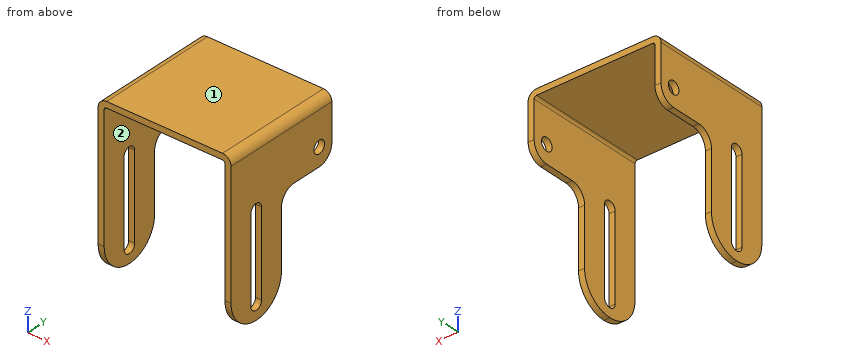
```python
from build123d import *

# Parameters (mm, degrees)
BASE_FLANGE1_DEPTH = 40
SKETCH6_W          = 34
SKETCH6_H          = 20
CUT_EXTRUDE1_DEPTH = 79.993670633
FILLET1_R          = 10
FILLET2_R          = 5
SKETCH7_R          = 2.1
CUT_EXTRUDE2_DEPTH = 79.993670633


# Read off the part's stored shape, not the designer's step: Base-Flange1
with BuildPart() as part:
    # Base-Flange1 outline → Base-Flange1 (new body)
    with BuildSketch(Plane(origin=(0, 0, 0), x_dir=(1, 0, 0), z_dir=(0, 1, 0))):
        with BuildLine():
            Line((-20, 0.8), (-20, 52))
            Line((-20, 52), (-22, 52))
            Line((-22, 52), (-22, 0.8))
            ThreePointArc((-22, 0.8), (-21.179898987, -1.179898987), (-19.2, -2))
            Line((-19.2, -2), (19.2, -2))
            ThreePointArc((19.2, -2), (21.179898987, -1.179898987), (22, 0.8))
            Line((22, 0.8), (22, 52))
            Line((22, 52), (20, 52))
            Line((20, 52), (20, 0.8))
            ThreePointArc((20, 0.8), (19.765685425, 0.234314575), (19.2, 0))
            Line((19.2, 0), (-19.2, 0))
            ThreePointArc((-19.2, 0), (-19.765685425, 0.234314575), (-20, 0.8))
        make_face()
    extrude(amount=BASE_FLANGE1_DEPTH)

    # Sketch6 → Cut-Extrude1 (cut, through all)
    with BuildSketch(Plane(origin=(22, 0, 0), x_dir=(0, 0, -1), z_dir=(1, 0, 0))):
        with Locations((35, 30)):
            Rectangle(SKETCH6_W, SKETCH6_H)
    extrude(amount=-CUT_EXTRUDE1_DEPTH, mode=Mode.SUBTRACT)

    # Fillet1
    fillet1_edges = [part.edges().sort_by_distance(p)[0] for p in [
        (-21, 0, -52),
        (-21, 20, -52),
        (21, 0, -52),
        (21, 20, -52),
    ]]
    fillet(fillet1_edges, radius=FILLET1_R - 0.0001)  # a hair under: the kernel refuses the full size

    # Fillet2
    fillet2_edges = [part.edges().sort_by_distance(p)[0] for p in [
        (-21, 40, -18),
        (21, 40, -18),
        (-21, 20, -18),
        (21, 20, -18),
    ]]
    fillet(fillet2_edges, radius=FILLET2_R)

    # Sketch7 → Cut-Extrude2 (cut, through all)
    with BuildSketch(Plane(origin=(22, 0, 0), x_dir=(0, 0, -1), z_dir=(1, 0, 0))):
        with Locations((12, 35)):
            Circle(SKETCH7_R)
        with BuildLine():
            Line((18.9, 12.1), (46.9, 12.1))
            ThreePointArc((46.9, 12.1), (49, 10), (46.9, 7.9))
            Line((46.9, 7.9), (18.9, 7.9))
            ThreePointArc((18.9, 7.9), (16.8, 10), (18.9, 12.1))
        make_face()
    extrude(amount=-CUT_EXTRUDE2_DEPTH, mode=Mode.SUBTRACT)


solid = part.part
```
Check sheet for the modelled part. Datum: model origin and axes. Units: mm. Face numbers are marked on the shaded views. A direction names the side the tool comes from. Coordinates: 2 decimals unless noted, no trailing zeros. Write each loop counter-clockwise with the first axis right and the second up, starting at its lowest first coordinate (ties: lowest second). Pieces come first, ordered by that corner, then holes. Notation, with made-up numbers: (-34.5, 45) -> (-29.5, 45) arc R9 cw to (-29.5, 59) -> close; hole circle Ø6 at (2, 66). An arc over 180 degrees is marked (long way). Use a Markdown table: item, result.
1. Scan lines: line 1 along Y through (x, z) = (-21, -12); line 2 along X through (y, z) = (22, -14.5); line 3 along Z through (x, y) = (16, 32.5). Record each from-to range of solid material in increasing order.
Reported:
| item | result |
|---|---|
| line 1 | y = 0 to 32.9, 37.1 to 40 |
| line 2 | x = -22 to -20, 20 to 22 |
| line 3 | z = 0 to 2 |
2. Sectioned sample at B-B (y = 4). Enter the section's corners in (x, z).
Reported:
| item | result |
|---|---|
| outline | (-22, -50) -> (-20, -50) -> (-20, -0.8) arc R0.8 cw to (-19.2, 0) -> (19.2, 0) arc R0.8 cw to (20, -0.8) -> (20, -50) -> (22, -50) -> (22, -0.8) arc R2.8 ccw to (19.2, 2) -> (-19.2, 2) arc R2.8 ccw to (-22, -0.8) -> close |
3. Sectioned sample at C-C (z = -31). Enter the section's corners in (x, y).
Reported:
| item | result |
|---|---|
| outline | (-22, 0) -> (-20, 0) -> (-20, 7.9) -> (-22, 7.9) -> close; (-22, 12.1) -> (-20, 12.1) -> (-20, 20) -> (-22, 20) -> close; (20, 0) -> (22, 0) -> (22, 7.9) -> (20, 7.9) -> close; (20, 12.1) -> (22, 12.1) -> (22, 20) -> (20, 20) -> close |
4. Sectioned sample at A-A (z = -12). Enter the section's corners in (x, y).
Reported:
| item | result |
|---|---|
| outline | (-22, 0) -> (-20, 0) -> (-20, 32.9) -> (-22, 32.9) -> close; (-22, 37.1) -> (-20, 37.1) -> (-20, 40) -> (-22, 40) -> close; (20, 0) -> (22, 0) -> (22, 32.9) -> (20, 32.9) -> close; (20, 37.1) -> (22, 37.1) -> (22, 40) -> (20, 40) -> close |
5. Go/stop test with flat-tipped pins: pin 1 Ø0.6 at (x, z) = (20.5, -30.5) entering from +Y; pin 2 Ø5 at (y, z) = (35, -12) entering from -X; pin 3 Ø0.6 at (x, y) = (-21, 29.5) entering from -Z; pin 4 Ø2.5 at (y, z) = (35, -12) entering from -X. Record where each tip stops, or that it passes through.
Reported:
| item | result |
|---|---|
| pin 1 | stops at y = 20 |
| pin 2 | stops at x = -22 |
| pin 3 | stops at z = -18 |
| pin 4 | passes through |
6. Tool access check on the marked faces 1 and 2. Record the directions out of +Z, -Z, +X, -X, +Y, -Y that give a thin tool (end or side, any length) a straight path to the whole face; none if there is none.
Reported:
| item | result |
|---|---|
| face 1 | +Z, +X, -X, +Y, -Y |
| face 2 | -Z, +Y, -Y |
7. Sectioned sample at D-D (x = -1.5). Enter the section's corners in (y, z), plus the area to 3 significant figures.
Reported:
| item | result |
|---|---|
| outline | (0, 0) -> (40, 0) -> (40, 2) -> (0, 2) -> close |
| area | 80.0 mm2 |
